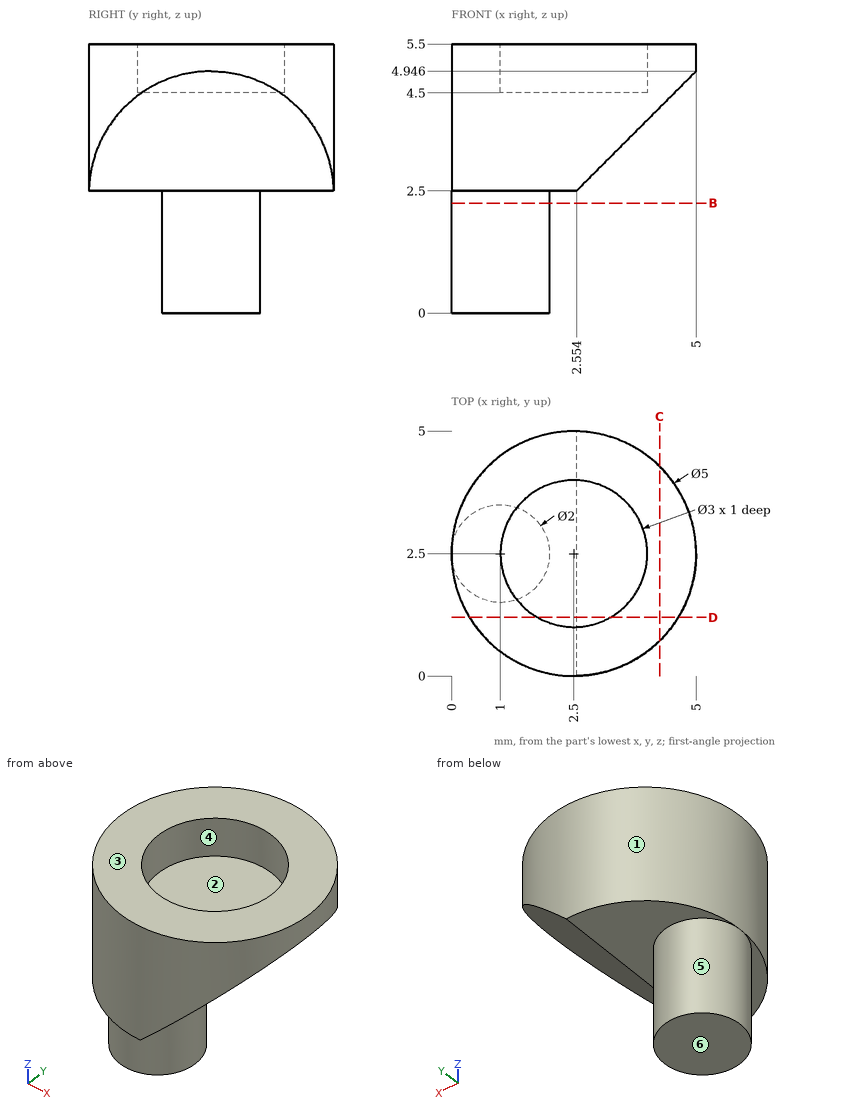
Design review of the part shown in the three views and the two pictorial views. Dimensions are in mm from the part's minimum x, y and z. A direction names the side the tool comes from. Round coordinates to 2 decimals unless told otherwise and drop trailing zeros. Loops run counter-clockwise (first coordinate to the right, second up) from the corner with the lowest first, then second, coordinate; pieces in that order, holes last.
(1) We need section D-D (y = 1.2). Give the boundary of the cut face in (x, z) (1 decimal).
Returned:
outline: (0.4, 2.5) - (2.6, 2.5) - (4.6, 4.6) - (4.6, 5.5) - (3.2, 5.5) - (3.2, 4.5) - (1.8, 4.5) - (1.8, 5.5) - (0.4, 5.5) - close
(2) Wall thickness on line 1 along Y through (x, z) = (2.5, 5.1); line 2 along Z through (x, y) = (2.1, 4.7); line 3 along Z through (x, y) = (1.45, 1.5): over which ranges is each line inside the solid? List them lowest first.
Returned:
line 1: y = 0 to 1, 4 to 5
line 2: z = 2.5 to 5.5
line 3: z = 2.5 to 4.5
(3) Tool access review of the marked faces 4, 5 and 6: name each direction out of +Z, -Z, +X, -X, +Y, -Y from which nothing blocks a thin tool from reaching the whole face with its end or side.
Returned:
face 4: +Z
face 5: -Z
face 6: -Z, +X, -X, +Y, -Y
(4) Clearance check with flat-ended pins moving along their axes: P1, Ø0.9, axis at x = 2, y = 3, coming from the +Z side; P2, Ø1.5, axis at y = 3.5, z = 1, coming from the +X side; P3, Ø1.5, axis at y = 1, z = 2, coming from the +X side (1 decimal). State where each tip first meets the part, or that it passes through.
Returned:
P1: stops at z = 4.5
P2: stops at x = 1.97
P3: stops at x = 2.8
(5) We need section B-B (z = 2.25). Give the boundary of the cut face in (x, y).
Returned:
outline: circle Ø2 at (1, 2.5)
(6) We need section C-C (x = 4.25). Give the boundary of the cut face in (y, z) (1 decimal).
Returned:
outline: (0.7, 4.2) - (4.3, 4.2) - (4.3, 5.5) - (0.7, 5.5) - close
(7) Mouldability with a two-part tool opening along Y and no side actions: class the marked faces 1, 2 and 3 as released by +Y, released by -Y, zero draft, split by the parting line, or undercut.
Returned:
face 1: split by the parting line
face 2: undercut
face 3: zero draft
